```python
from build123d import *

# Parameters (mm, degrees)
SKETCH1_W           = 101.6
SKETCH1_H           = 38.1
BOSS_EXTRUDE1_DEPTH = 4.2926
FILLET1_R           = 2.54
SKETCH2_W           = 4.2926
SKETCH2_H           = 19.05
CUT_EXTRUDE1_DEPTH  = 4.2926
FILLET2_R           = 1.905
FILLET3_R           = 1.27


with BuildPart() as part:
    # Sketch1 → Boss-Extrude1 (new body)
    with BuildSketch(Plane.XY):
        Rectangle(SKETCH1_W, SKETCH1_H)
    extrude(amount=BOSS_EXTRUDE1_DEPTH)

    # Fillet1
    fillet1_edges = [part.edges().sort_by_distance(p)[0] for p in [
        (50.8, -19.05, 2.1463),
        (-50.8, -19.05, 2.1463),
        (-50.8, 19.05, 2.1463),
        (50.8, 19.05, 2.1463),
    ]]
    fillet(fillet1_edges, radius=FILLET1_R)

    # Sketch2 → Cut-Extrude1 (cut)
    with BuildSketch(Plane.XY.offset(4.2926)):
        with Locations((-41.91, 9.525)):
            Rectangle(SKETCH2_W, SKETCH2_H)
        with Locations((-27.94, 9.525)):
            Rectangle(SKETCH2_W, SKETCH2_H)
        with Locations((-11.43, 9.525)):
            Rectangle(SKETCH2_W, SKETCH2_H)
        with Locations((11.43, 9.525)):
            Rectangle(SKETCH2_W, SKETCH2_H)
        with Locations((27.94, 9.525)):
            Rectangle(SKETCH2_W, SKETCH2_H)
        with Locations((41.91, 9.525)):
            Rectangle(SKETCH2_W, SKETCH2_H)
    extrude(amount=-CUT_EXTRUDE1_DEPTH, mode=Mode.SUBTRACT)

    # Fillet2
    fillet2_edges = [part.edges().sort_by_distance(p)[0] for p in [
        (-39.7637, 19.05, 2.1463),
        (-44.0563, 19.05, 2.1463),
        (-25.7937, 19.05, 2.1463),
        (-30.0863, 19.05, 2.1463),
        (-9.2837, 19.05, 2.1463),
        (-13.5763, 19.05, 2.1463),
        (13.5763, 19.05, 2.1463),
        (9.2837, 19.05, 2.1463),
        (30.0863, 19.05, 2.1463),
        (25.7937, 19.05, 2.1463),
        (44.0563, 19.05, 2.1463),
        (39.7637, 19.05, 2.1463),
    ]]
    fillet(fillet2_edges, radius=FILLET2_R)

    # Fillet3
    fillet3_edges = [part.edges().sort_by_distance(p)[0] for p in [
        (-39.7637, 0, 2.1463),
        (-44.0563, 0, 2.1463),
        (-25.7937, 0, 2.1463),
        (-30.0863, 0, 2.1463),
        (-9.2837, 0, 2.1463),
        (-13.5763, 0, 2.1463),
        (13.5763, 0, 2.1463),
        (9.2837, 0, 2.1463),
        (30.0863, 0, 2.1463),
        (25.7937, 0, 2.1463),
        (44.0563, 0, 2.1463),
        (39.7637, 0, 2.1463),
    ]]
    fillet(fillet3_edges, radius=FILLET3_R)


solid = part.part
```
Part model, mm, in its own coordinate system. A direction names the side the tool comes from. Round coordinates to 2 decimals unless told otherwise and drop trailing zeros. Loops run counter-clockwise (first coordinate to the right, second up) from the corner with the lowest first, then second, coordinate; pieces in that order, holes last. Notation, with made-up numbers: (46, 33.25) -> (97, 33.25) arc R24 cw to (97, 58.25) -> close; hole circle Ø7 at (64, -26.75). An arc over 180 degrees is marked (long way). Use CSV: the item, a comma, the result in double quotes. Start each with the question number.
1) Pull direction X, two halves, no side cores. Call faces 3 (the flat face through (25.794, 9, 2)), 4 (the cylindrical face through (50.076, 18.286, 2.176)), 5 (the flat face through (0, 19.05, 2)): +X half, -X half, draft (parallel to the pull), parting line (faces both ways), or undercut.
2) Wall check: L1, parallel to Y at x = 11, z = 1.9; L2, parallel to Y at x = 29.5, z = 2.65. Give the ranges that are in metal, low to high. Write a range as [from, to].
3) Drop flat-ended pins along their axis: P1, Ø0.5, axis at x = -42, z = 1.5, coming from the +Y side; P2, Ø1.9, axis at x = -11, z = 3, coming from the +Y side; P3, Ø1, axis at x = -31, z = 3, coming from the +Y side. Give the stop position or say it passes through.
4) Cut at A-A, the plane y = 9. Write the cut outline in (x, z), plus the area to 3 significant figures.
5) Which spindle directions (+Z, -Z, +X, -X, +Y, -Y) get a long thin tool onto all of the face, cutting with end or side? Do faces 1 (the flat face through (-30.086, 9, 2)), 2 (the flat face through (-35, 19.05, 2)). Say none if no direction does.
Determined:
1,face 3,"undercut"
1,face 4,"+X half"
1,face 5,"draft"
2,L1,"y = [-19.05, 0]"
2,L2,"y = [-19.05, 0.2]"
3,P1,"stops at y = 0"
3,P2,"stops at y = 0.1"
3,P3,"stops at y = 18.99"
4,outline,"(-50.8, 0) -> (-44.06, 0) -> (-44.06, 4.29) -> (-50.8, 4.29) -> close; (-39.76, 0) -> (-30.09, 0) -> (-30.09, 4.29) -> (-39.76, 4.29) -> close; (-25.79, 0) -> (-13.58, 0) -> (-13.58, 4.29) -> (-25.79, 4.29) -> close; (-9.28, 0) -> (9.28, 0) -> (9.28, 4.29) -> (-9.28, 4.29) -> close; (13.58, 0) -> (25.79, 0) -> (25.79, 4.29) -> (13.58, 4.29) -> close; (30.09, 0) -> (39.76, 0) -> (39.76, 4.29) -> (30.09, 4.29) -> close; (44.06, 0) -> (50.8, 0) -> (50.8, 4.29) -> (44.06, 4.29) -> close"
4,area,"326 mm2"
5,face 1,"+Z, -Z, +Y"
5,face 2,"+Z, -Z, +X, -X, +Y"
